Part model, mm, in its own coordinate system. A direction names the side the tool comes from. Coordinates: 2 decimals unless noted, no trailing zeros. Order: outer loops, then holes, each group sorted by start corner. A loop starts at its lowest first (then second) coordinate and runs counter-clockwise, first axis right, second up.
from build123d import *

# Parameters (mm, degrees)
SKETCH1_R           = 2
BOSS_EXTRUDE1_DEPTH = 2


with BuildPart() as part:
    # Sketch1 → Boss-Extrude1 (new body)
    with BuildSketch(Plane(origin=(0, 0, 0), x_dir=(1, 0, 0), z_dir=(0, 1, 0))):
        with BuildLine():
            Line((165.082783055, -24.990305924), (165.082783055, 3.009694076))
            Line((165.082783055, 3.009694076), (129.082783055, 3.009694076))
            ThreePointArc((129.082783055, 3.009694076), (123.082783055, 9.009694076), (117.082783055, 3.009694076))
            Line((117.082783055, 3.009694076), (81.082783055, 3.009694076))
            Line((81.082783055, 3.009694076), (81.082783055, -24.990305924))
            Line((81.082783055, -24.990305924), (117.082783055, -24.990305924))
            ThreePointArc((117.082783055, -24.990305924), (123.082783055, -30.990305924), (129.082783055, -24.990305924))
            Line((129.082783055, -24.990305924), (165.082783055, -24.990305924))
        make_face()
        with Locations(Location((123.082783055, 5.009694076, 0), (0, 0, 270))):
            Circle(SKETCH1_R, mode=Mode.SUBTRACT)
        with Locations(Location((123.082783055, -26.990305924, 0), (0, 0, 270))):
            Circle(SKETCH1_R, mode=Mode.SUBTRACT)
    extrude(amount=BOSS_EXTRUDE1_DEPTH)


solid = part.part
Q1. Mould opens along Z. For faces 1 (the face through (121.13, 0.99, -5.44)), 2 (the face through (122, 0, 11)), 3 (the face through (99, 1, 24.99)) say: pulls with the +Z half, pulls with the -Z half, needs draft (parallel to the pull), parting line crosses it, or undercut.
Results list:
face 1: undercut
face 2: needs draft
face 3: pulls with the +Z half
Q2. Cut at A-A on z = 28. Write the cut outline in (x, y).
Results list:
outline: (117.89, 0) - (121.36, 0) - (121.36, 2) - (117.89, 2) - close; (124.81, 0) - (128.27, 0) - (128.27, 2) - (124.81, 2) - close
Q3. Cut at D-D on x = 143.5. Write the cut outline in (y, z), and give its area (3 significant figures).
Results list:
outline: (0, -3.01) - (2, -3.01) - (2, 24.99) - (0, 24.99) - close
area: 56.0 mm2
Q4. Cut at B-B on y = 0.7. Write the cut outline in (x, z), and give its area (3 significant figures).
Results list:
outline: (81.08, -3.01) - (117.08, -3.01) arc R6 ccw to (129.08, -3.01) - (165.08, -3.01) - (165.08, 24.99) - (129.08, 24.99) arc R6 ccw to (117.08, 24.99) - (81.08, 24.99) - close; hole circle Ø4 at (123.08, -5.01); hole circle Ø4 at (123.08, 26.99)
area: 2,440 mm2
Q5. Wall check: line 1 along Z through (x, y) = (147, 0.9); line 2 along Z through (x, y) = (126, 0.4). Give the ranges that are in metal, low to high.
Results list:
line 1: z = -3.01 to 24.99
line 2: z = -8.25 to 30.23
Q6. Which spindle directions (+Z, -Z, +X, -X, +Y, -Y) get a long thin tool onto all of the face, cutting with end or side? Do faces 4 (the face through (147, 1, -3.01)), 5 (the face through (99, 1, -3.01)), 6 (the face through (147, 1, 24.99)). Say none if no direction does.
Results list:
face 4: -Z, +X, +Y, -Y
face 5: -Z, -X, +Y, -Y
face 6: +Z, +X, +Y, -Y
Q7. Cut at C-C on x = 124. Write the cut outline in (y, z).
Results list:
outline: (0, -8.94) - (2, -8.94) - (2, -6.79) - (0, -6.79) - close; (0, -3.23) - (2, -3.23) - (2, 25.21) - (0, 25.21) - close; (0, 28.77) - (2, 28.77) - (2, 30.92) - (0, 30.92) - close
Q8. Pin check, flat tip, straight feed: pin 1 Ø0.6 at (x, y) = (143.5, 0.5) entering from -Z. Stop position of the tip, or through.
Results list:
pin 1: stops at z = -3.01
